Read the model definition and answer for the solid it produces. Units are mm, in the model's axes. A direction names the side the tool comes from. Coordinates: 2 decimals unless noted, no trailing zeros. Loops run counter-clockwise (first coordinate to the right, second up) from the corner with the lowest first, then second, coordinate; pieces in that order, holes last.
Q1. Which of the six approach directions +Z, -Z, +X, -X, +Y, -Y give full straight-line access (tool end or side, diameter ignored) to faces 1 (the face through (68.03, -0.18, 63.91)), 2 (the face through (95.952, -19, 79)), 3 (the face through (1, 31, 19.705))?
Q2. Section B-B (x = 100) is taken. Give the vertices of the cut face in (y, z), then the cut area to 3 significant figures.
Q3. Straight lines are drawn through the part: line 1 (X direction, y = -15, z = -10); line 2 (Z direction, x = 13.5, y = -10.5); line 3 (Y direction, x = 41, z = 78). For each, find the intervals that lie inside material, in ascending order.
Q4. Section A-A (z = -7.5) is taken. Give the vertices of the cut face in (x, y).
Q5. The mould has two halves that part along Z. Classify faces 4 (the face through (-1, -38.1, 0)), 5 (the face through (56.652, -19, 36)), 6 (the face through (112, 0, 84.244)), 7 (the face through (92, 12.7, 69)): pulls with the +Z half, pulls with the -Z half, needs draft (parallel to the pull), parting line crosses it, or undercut.
Q6. Flat-ended cylindrical pins translate along their axes: P1, Ø6, axis at y = 22.5, z = 57, coming from the +X side; P2, Ø1, axis at x = 65.5, y = 0, coming from the +Z side; P3, Ø6.5, axis at x = 84.5, y = -22, coming from the -Z side. Find the tip coordinate at first contact, or state that the pin passes through.
from build123d import *

# Parameters (mm, degrees)
F1_DEPTH = 38.1
F2_DEPTH = 25.4
F3_DEPTH = 12.7
F4_DEPTH = 12.7
F5_R     = 5.08


with BuildPart() as f1:
    # F0 (on Front) → F1 (new body, symmetric)
    with BuildSketch(Plane.XZ):
        Polygon((-63.397139, 19.704513), (-63.397139, -19.704513), (63.397139, -19.704513), (63.397139, 19.704513), (56.652256, 19.704513), align=None)
    extrude(amount=F1_DEPTH, both=True)

    # F0 (on Front) → F2 (join, symmetric)
    with BuildSketch(Plane.XZ):
        with BuildLine():
            add(Edge.make_bspline(
                [(-63.397139, 19.704513), (-5.140318, 19.704513), (22.56023, 108.517617), (95.952414, 84.243942)],
                knots=[0, 0, 0, 0, 171.923291, 171.923291, 171.923291, 171.923291], degree=3))
            Line((-63.397139, 19.704513), (56.652256, 19.704513))
            Line((56.652256, 19.704513), (56.652256, 53.116519))
            ThreePointArc((56.652256, 53.116519), (63.466087, 68.877623), (79.615708, 74.711181))
            Line((79.615708, 74.711181), (95.952414, 74.711181))
            Line((95.952414, 74.711181), (95.952414, 84.243942))
        make_face()
    extrude(amount=F2_DEPTH, both=True)

    # F0 (on Front) → F3 (join, symmetric)
    with BuildSketch(Plane.XZ):
        with BuildLine():
            Line((56.652256, 19.704513), (63.397139, 19.704513))
            Line((63.397139, 19.704513), (63.397139, 53.116519))
            ThreePointArc((63.397139, 53.116519), (68.1554, 64.028229), (79.389192, 67.966297))
            Line((79.389192, 67.966297), (95.952414, 67.966297))
            Line((95.952414, 67.966297), (95.952414, 74.711181))
            Line((95.952414, 74.711181), (79.615708, 74.711181))
            ThreePointArc((79.615708, 74.711181), (63.466087, 68.877623), (56.652256, 53.116519))
            Line((56.652256, 53.116519), (56.652256, 19.704513))
        make_face()
    extrude(amount=F3_DEPTH, both=True)

    # F0 (on Front) → F4 (join, symmetric)
    with BuildSketch(Plane.XZ):
        Polygon((128.507696, 84.243942), (95.952414, 84.243942), (95.952414, 74.711181), (95.952414, 67.966297), (95.952414, 63.923942), (128.507696, 63.923942), align=None)
    extrude(amount=F4_DEPTH, both=True)

    # F5
    f5_edges = [f1.edges().sort_by_distance(p)[0] for p in [
        (-63.397139, -38.1, 0),
        (63.397139, -38.1, 0),
        (63.397139, 38.1, 0),
        (-63.397139, 38.1, 0),
    ]]
    fillet(f5_edges, radius=F5_R)


solid = f1.part
Numbers:
1. face 1: -Z, +Y, -Y
1. face 2: +Z, -Z, +X, -Y
1. face 3: +X, +Y
2. outline: (-12.7, 63.92) - (12.7, 63.92) - (12.7, 84.24) - (-12.7, 84.24) - close
2. area: 516 mm2
3. line 1: x = -63.4 to 63.4
3. line 2: z = -19.7 to 63.43
3. line 3: y = -25.4 to 25.4
4. outline: (-63.4, -33.02) arc R5.08 ccw to (-58.32, -38.1) - (58.32, -38.1) arc R5.08 ccw to (63.4, -33.02) - (63.4, 33.02) arc R5.08 ccw to (58.32, 38.1) - (-58.32, 38.1) arc R5.08 ccw to (-63.4, 33.02) - close
5. face 4: needs draft
5. face 5: undercut
5. face 6: pulls with the +Z half
5. face 7: undercut
6. P1: stops at x = 57.78
6. P2: stops at z = 88.24
6. P3: stops at z = 74.71
